```python
from build123d import *

# Parameters (mm, degrees)
BOSS_EXTRUDE1_DEPTH      = 6.35
FILLET1_R                = 5.08
SKETCH3_W                = 277.368
SKETCH3_H                = 25.4
BOSS_EXTRUDE2_DEPTH      = 3.175
SKETCH5_W                = 277.368
SKETCH5_H                = 25.4
BOSS_EXTRUDE3_DEPTH      = 3.175
BOSS_EXTRUDE4_DEPTH      = 1.5875
BOSS_EXTRUDE4_DEPTH_BACK = 1.5875
BOSS_EXTRUDE5_DEPTH      = 1.5875
BOSS_EXTRUDE5_DEPTH_BACK = 1.5875
BOSS_EXTRUDE6_DEPTH      = 1.5875
BOSS_EXTRUDE6_DEPTH_BACK = 1.5875
BOSS_EXTRUDE7_DEPTH      = 1.5875
BOSS_EXTRUDE7_DEPTH_BACK = 1.5875
BOSS_EXTRUDE8_DEPTH      = 1.5875
BOSS_EXTRUDE8_DEPTH_BACK = 1.5875
BOSS_EXTRUDE9_DEPTH      = 1.5875
BOSS_EXTRUDE9_DEPTH_BACK = 1.5875


with BuildPart() as part:
    # Sketch2 → Boss-Extrude1 (new body)
    with BuildSketch(Plane.XY):
        with BuildLine():
            Line((-5.12438972, 14.653837172), (267.16361028, 14.653837172))
            ThreePointArc((267.16361028, 14.653837172), (268.959661504, 15.397785947), (269.70361028, 17.193837172))
            Line((269.70361028, 17.193837172), (269.70361028, 75.613837172))
            ThreePointArc((269.70361028, 75.613837172), (268.959661504, 77.409888396), (267.16361028, 78.153837172))
            Line((267.16361028, 78.153837172), (-5.12438972, 78.153837172))
            ThreePointArc((-5.12438972, 78.153837172), (-6.920440944, 77.409888396), (-7.66438972, 75.613837172))
            Line((-7.66438972, 75.613837172), (-7.66438972, 17.193837172))
            ThreePointArc((-7.66438972, 17.193837172), (-6.920440944, 15.397785947), (-5.12438972, 14.653837172))
        make_face()
        Polygon((30.05461028, 24.406794359), (4.65461028, 68.400884872), (55.45461028, 68.400884872), align=None, mode=Mode.SUBTRACT)
        Polygon((70.44061028, 68.400882428), (95.84061028, 24.406791915), (45.04061028, 24.406791915), align=None, mode=Mode.SUBTRACT)
        Polygon((110.82627023, 24.305837172), (85.42627023, 68.299927684), (136.22627023, 68.299927684), align=None, mode=Mode.SUBTRACT)
        Polygon((125.81227023, 24.305834728), (151.21227023, 68.29992524), (176.61227023, 24.305834728), align=None, mode=Mode.SUBTRACT)
        Polygon((191.59793018, 24.204879984), (166.19793018, 68.198970496), (216.99793018, 68.198970496), align=None, mode=Mode.SUBTRACT)
        Polygon((206.58393018, 24.20487754), (231.98393018, 68.198968052), (257.38393018, 24.20487754), align=None, mode=Mode.SUBTRACT)
    extrude(amount=BOSS_EXTRUDE1_DEPTH)

    # Fillet1
    fillet1_edges = [part.edges().sort_by_distance(p)[0] for p in [
        (257.38393018, 24.20487754, 3.175),
        (231.98393018, 68.198968052, 3.175),
        (206.58393018, 24.20487754, 3.175),
        (176.61227023, 24.305834728, 3.175),
        (151.21227023, 68.29992524, 3.175),
        (125.81227023, 24.305834728, 3.175),
        (4.65461028, 68.400884872, 3.175),
        (30.05461028, 24.406794359, 3.175),
        (55.45461028, 68.400884872, 3.175),
        (95.84061028, 24.406791915, 3.175),
        (70.44061028, 68.400882428, 3.175),
        (45.04061028, 24.406791915, 3.175),
        (85.42627023, 68.299927684, 3.175),
        (110.82627023, 24.305837172, 3.175),
        (136.22627023, 68.299927684, 3.175),
        (166.19793018, 68.198970496, 3.175),
        (191.59793018, 24.204879984, 3.175),
        (216.99793018, 68.198970496, 3.175),
    ]]
    fillet(fillet1_edges, radius=FILLET1_R)

    # Sketch3 → Boss-Extrude2 (add)
    with BuildSketch(Plane(origin=(0, 78.153837172, 0), x_dir=(1, 0, 0), z_dir=(0, 1, 0))):
        with Locations((131.01961028, -12.7)):
            Rectangle(SKETCH3_W, SKETCH3_H)
    extrude(amount=-BOSS_EXTRUDE2_DEPTH)

    # Sketch5 → Boss-Extrude3 (add)
    with BuildSketch(Plane(origin=(0, 14.653837172, 0), x_dir=(-1, 0, 0), z_dir=(0, -1, 0))):
        with Locations((-131.01961028, -12.7)):
            Rectangle(SKETCH5_W, SKETCH5_H)
    extrude(amount=-BOSS_EXTRUDE3_DEPTH)

    # Sketch8 → Boss-Extrude4 (add, two sides: drawn at the far end of the back side and taken through both)
    with BuildSketch(Plane(origin=(43.13561028, 0, 0), x_dir=(0, 0, -1), z_dir=(1, 0, 0)).offset(-BOSS_EXTRUDE4_DEPTH_BACK)):
        Polygon((-25.4, 17.828837172), (-6.35, 17.828837172), (-6.35, 36.878837172), align=None)
    extrude(amount=BOSS_EXTRUDE4_DEPTH + BOSS_EXTRUDE4_DEPTH_BACK)

    # Sketch9 → Boss-Extrude5 (add, two sides: drawn at the far end of the back side and taken through both)
    with BuildSketch(Plane(origin=(124.41561028, 0, 0), x_dir=(0, 0, -1), z_dir=(1, 0, 0)).offset(-BOSS_EXTRUDE5_DEPTH_BACK)):
        Polygon((-25.4, 17.828837172), (-6.35, 17.828837172), (-6.35, 36.878837172), align=None)
    extrude(amount=BOSS_EXTRUDE5_DEPTH + BOSS_EXTRUDE5_DEPTH_BACK)

    # Sketch10 → Boss-Extrude6 (add, two sides: drawn at the far end of the back side and taken through both)
    with BuildSketch(Plane(origin=(205.69561028, 0, 0), x_dir=(0, 0, -1), z_dir=(1, 0, 0)).offset(-BOSS_EXTRUDE6_DEPTH_BACK)):
        Polygon((-25.4, 17.828837172), (-6.35, 17.828837172), (-6.35, 36.878837172), align=None)
    extrude(amount=BOSS_EXTRUDE6_DEPTH + BOSS_EXTRUDE6_DEPTH_BACK)

    # Sketch11 → Boss-Extrude7 (add, two sides: drawn at the far end of the back side and taken through both)
    with BuildSketch(Plane.ZY.offset(-218.133612998).offset(-BOSS_EXTRUDE7_DEPTH_BACK)):
        Polygon((25.4, 74.978837172), (6.35, 74.978837172), (6.35, 55.928837172), align=None)
    extrude(amount=BOSS_EXTRUDE7_DEPTH + BOSS_EXTRUDE7_DEPTH_BACK)

    # Sketch12 → Boss-Extrude8 (add, two sides: drawn at the far end of the back side and taken through both)
    with BuildSketch(Plane.ZY.offset(-135.652884913).offset(-BOSS_EXTRUDE8_DEPTH_BACK)):
        Polygon((25.4, 74.978837172), (6.35, 74.978837172), (6.35, 55.928837172), align=None)
    extrude(amount=BOSS_EXTRUDE8_DEPTH + BOSS_EXTRUDE8_DEPTH_BACK)

    # Sketch13 → Boss-Extrude9 (add, two sides: drawn at the far end of the back side and taken through both)
    with BuildSketch(Plane.ZY.offset(-54.372884913).offset(-BOSS_EXTRUDE9_DEPTH_BACK)):
        Polygon((25.4, 74.978837172), (6.35, 74.978837172), (6.35, 55.928837172), align=None)
    extrude(amount=BOSS_EXTRUDE9_DEPTH + BOSS_EXTRUDE9_DEPTH_BACK)


solid = part.part
```
For this review, take the finished solid that the model builds, in its own axes (mm). A direction names the side the tool comes from. Coordinates: 2 decimals unless noted, no trailing zeros. Write each loop counter-clockwise with the first axis right and the second up, starting at its lowest first coordinate (ties: lowest second). Pieces come first, ordered by that corner, then holes. Notation, with made-up numbers: (54, 86) - (59, 86) arc R27 ccw to (59, 114) - close; hole circle Ø3 at (19, 4.5). An arc over 180 degrees is marked (long way). Answer in a Markdown table with one row per item. Add a question column.
Q1. Tool access review of faces 5 (the flat face through (84, 17.829, 16)), 6 (the flat face through (52.785, 68, 14)), 7 (the flat face through (43.11, 27.49, 15.74)): name each direction out of +Z, -Z, +X, -X, +Y, -Y from which nothing blocks a thin tool from reaching the whole face with its end or side.
Q2. We need section B-B, the plane x = 179.5. State the section outline as (y, z) points.
Q3. We need section D-D, the plane x = 62. State the section outline as (y, z) points.
Q4. Draft analysis for pull direction X (two halves, no side actions). For faces 1 (the cylindrical face through (30.129, 29.487, 3.219)), 2 (the flat face through (207.283, 23, 12)), 3 (the flat face through (41.548, 23, 12)), 4 (the flat face through (239, 17.829, 16)), state which applies: +X half, -X half, draft (parallel to the pull), parting line (faces both ways), or undercut.
Q5. For probe 1 along X at (y, z) = (66.5, 6.5); probe 2 along X at (y, z) = (27, 13.5); probe 3 along Y at (x, z) = (90, 18), list the stretches that pass through material, from the lowest coordinate up.
Q6. We need section C-C, the plane y = 40.5. State the section outline as (x, z) points.
Q7. For P1, Ø15, axis at y = 32, z = 19, coming from the -X side; P2, Ø3, axis at x = 50.5, y = 28, coming from the +Z side, all flat-tipped, find the tip position at first contact; note any pin that passes through.
Answer list:
| question | item | result |
|---|---|---|
| 1 | face 5 | +Z |
| 1 | face 6 | +Z, -X |
| 1 | face 7 | +Z, +X, -X |
| 2 | outline | (14.65, 0) - (45.16, 0) - (45.16, 6.35) - (17.83, 6.35) - (17.83, 25.4) - (14.65, 25.4) - close; (68.2, 0) - (78.15, 0) - (78.15, 25.4) - (74.98, 25.4) - (74.98, 6.35) - (68.2, 6.35) - close |
| 3 | outline | (14.65, 0) - (24.41, 0) - (24.41, 6.35) - (17.83, 6.35) - (17.83, 25.4) - (14.65, 25.4) - close; (53.78, 0) - (78.15, 0) - (78.15, 25.4) - (74.98, 25.4) - (74.98, 6.35) - (53.78, 6.35) - close |
| 4 | face 1 | undercut |
| 4 | face 2 | +X half |
| 4 | face 3 | -X half |
| 4 | face 4 | draft |
| 5 | probe 1 | x = 52.79 to 55.96, 134.07 to 137.24, 216.55 to 219.72 |
| 5 | probe 2 | x = 41.55 to 44.72, 122.83 to 126, 204.11 to 207.28 |
| 5 | probe 3 | y = 14.65 to 17.83, 74.98 to 78.15 |
| 6 | outline | (-7.66, 0) - (20.76, 0) - (20.76, 6.35) - (-7.66, 6.35) - close; (39.35, 0) - (54.33, 0) - (54.33, 6.35) - (39.35, 6.35) - close; (86.55, 0) - (101.48, 0) - (101.48, 6.35) - (86.55, 6.35) - close; (120.18, 0) - (135.16, 0) - (135.16, 6.35) - (120.18, 6.35) - close; (167.26, 0) - (182.19, 0) - (182.19, 6.35) - (167.26, 6.35) - close; (201.01, 0) - (215.99, 0) - (215.99, 6.35) - (201.01, 6.35) - close; (247.98, 0) - (269.7, 0) - (269.7, 6.35) - (247.98, 6.35) - close |
| 7 | P1 | stops at x = 41.55 |
| 7 | P2 | stops at z = 6.35 |
